Study the drawing (mm; zero at the part's minimum x, y, z) and answer. A direction names the side the tool comes from. Coordinates: 2 decimals unless noted, no trailing zeros. Order: outer loops, then holes, each group sorted by start corner. A loop starts at its lowest first (then second) coordinate and runs counter-clockwise, first axis right, second up. Notation, with made-up numbers: (2, 31) -> (29, 31) arc R14 cw to (29, 35) -> close; hole circle Ø9 at (31, 37). An arc over 180 degrees is marked (long way). Put each result on its own line as item: value. Start each with the question number.
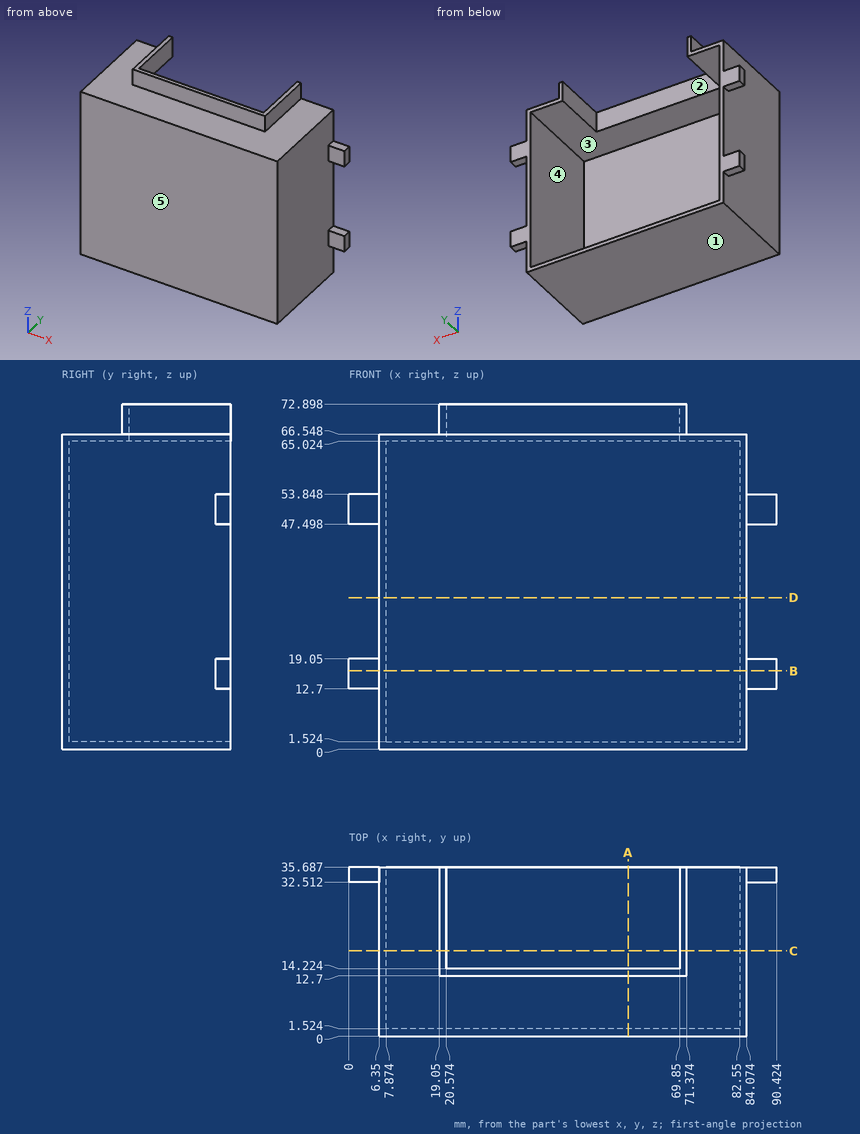
(1) Each of these flat-tipped pins is pushed along its axis until it touches: P1, Ø6.5, axis at y = 27.5, z = 68.5, coming from the +X side; P2, Ø6, axis at x = 18.5, z = 13, coming from the +Y side; P3, Ø3, axis at y = 23.5, z = 70.5, coming from the -X side. Where does it stop, or does it pass through?
(2) The part is cut by section B-B on z = 16.5. Determine the outline of the cut face in (x, y).
(3) The part is cut by section C-C on y = 18. Determine the outline of the cut face in (x, z), plus the area to 3 significant figures.
(4) Find the intervals of material crossed by L1, parallel to Z at x = 8, y = 20; L2, parallel to X at y = 32, z = 33.5; L3, parallel to Y at x = 15.5, z = 64, in increasing order.
(5) The part is cut by section A-A on x = 59. Determine the outline of the cut face in (y, z).
(6) For a pull along Z with two mould halves and no side action, classify the marked faces 1, 2 and 3 as released by +Z, released by -Z, zero draft, split by the parting line, or undercut.
(7) The part is cut by section D-D on z = 32. Determine the outline of the cut face in (x, y).
(8) A tool of negligible diameter and unlimited length cuts with its end or side. For the marked faces 4 and 5, from which of +Z, -Z, +X, -X, +Y, -Y can it reach the whole face along a straight path? Write none if from no direction.
Worked out:
1. P1: x = 84.07
1. P2: y = 1.52
1. P3: x = 19.05
2. outline: (0, 32.51) -> (6.35, 32.51) -> (6.35, 0) -> (84.07, 0) -> (84.07, 32.51) -> (90.42, 32.51) -> (90.42, 35.69) -> (82.55, 35.69) -> (82.55, 1.52) -> (7.87, 1.52) -> (7.87, 35.69) -> (0, 35.69) -> close
3. outline: (6.35, 0) -> (84.07, 0) -> (84.07, 66.55) -> (71.37, 66.55) -> (71.37, 72.9) -> (69.85, 72.9) -> (69.85, 65.02) -> (82.55, 65.02) -> (82.55, 1.52) -> (7.87, 1.52) -> (7.87, 65.02) -> (20.57, 65.02) -> (20.57, 72.9) -> (19.05, 72.9) -> (19.05, 66.55) -> (6.35, 66.55) -> close
3. area: 375 mm2
4. L1: 0 to 1.52, 65.02 to 66.55
4. L2: 6.35 to 7.87, 82.55 to 84.07
4. L3: 0 to 1.52
5. outline: (0, 0) -> (35.69, 0) -> (35.69, 1.52) -> (1.52, 1.52) -> (1.52, 65.02) -> (14.22, 65.02) -> (14.22, 72.9) -> (12.7, 72.9) -> (12.7, 66.55) -> (0, 66.55) -> close
6. face 1: released by -Z
6. face 2: zero draft
6. face 3: undercut
7. outline: (6.35, 0) -> (84.07, 0) -> (84.07, 35.69) -> (82.55, 35.69) -> (82.55, 1.52) -> (7.87, 1.52) -> (7.87, 35.69) -> (6.35, 35.69) -> close
8. face 4: +Y
8. face 5: +Z, -Z, +X, -X, -Y
